```python
from build123d import *

# Parameters (mm, degrees)
BOSS_EXTRUDE1_DEPTH = 5
CUT_EXTRUDE1_REACH  = 7
SKETCH3_W           = 5
SKETCH3_H           = 26.5


with BuildPart() as part:
    # Sketch2 → Boss-Extrude1 (new body)
    with BuildSketch(Plane.XY):
        Polygon((-50, 422.98), (-50, 0), (50, 0), (50, 422.98), (50, 493.000753821), align=None)
    extrude(amount=BOSS_EXTRUDE1_DEPTH)

    # Sketch3 → Cut-Extrude1 (cut, up to next)
    with BuildSketch(Plane.XY.offset(5), mode=Mode.PRIVATE) as cut_extrude1_sk1:
        with Locations((42.5, 325)):
            Rectangle(SKETCH3_W, SKETCH3_H)
    cut_extrude1_tool1 = extrude(cut_extrude1_sk1.sketch, amount=-CUT_EXTRUDE1_REACH, mode=Mode.PRIVATE) & part.part
    add(cut_extrude1_tool1.solids().sort_by_distance((42.5, 325, 5))[0], mode=Mode.SUBTRACT)


solid = part.part
```
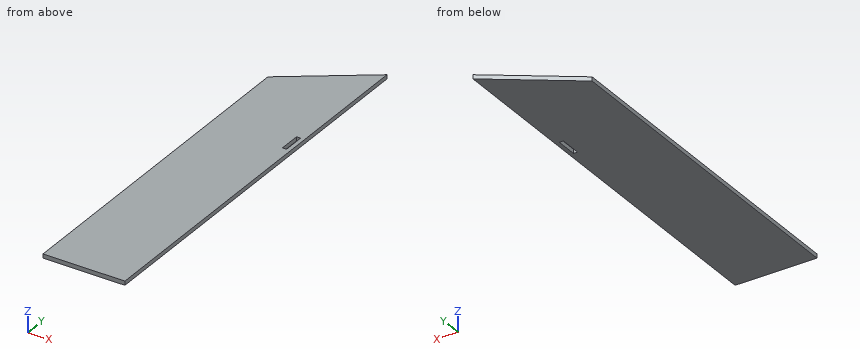
Could you check a few things on this model? Use its own coordinates, in mm. Give positions to 0.01 mm unless a question says otherwise; leave off trailing zeros. Loops run counter-clockwise (first coordinate to the right, second up) from the corner with the lowest first, then second, coordinate; pieces in that order, holes last. Notation, with made-up numbers: (22, 79.5) - (39, 79.5) arc R21 cw to (39, 90.5) - close; hole circle Ø5 at (24.25, -23). An arc over 180 degrees is marked (long way). Answer in a Markdown table with one row per item. Add a question column.
Q1. If we section it at A-A (y = 317.5): List the corners of the cut face in (x, z) for me.
Q2. If we section it at C-C (x = -32): List the corners of the cut face in (y, z) for me, plus the area to 3 significant figures.
Q3. If we section it at D-D (y = 444): List the corners of the cut face in (x, z) for me.
Q4. For pin 1 (8 mm diameter, centred on x = 34.5, y = 318.5, fed in from -Z); pin 2 (3 mm diameter, centred on x = -6, z = 3.5, fed in from +Y), each with a flat end and sliding along its axis, tell me the tip position at first contact or that it passes through.
Q5. If we section it at B-B (z = 3.85): List the corners of the cut face in (x, y) for me, plus the area to 3 significant figures.
Q6. Please list where these lines run through material, in increasing order: L1, parallel to X at y = 438, z = 1.75; L2, parallel to X at y = 469.5, z = 3.45; L3, parallel to Y at x = -4.5, z = 2.45. Write a range as from..to.
The answers:
| question | item | result |
|---|---|---|
| 1 | outline | (-50, 0) - (40, 0) - (40, 5) - (-50, 5) - close; (45, 0) - (50, 0) - (50, 5) - (45, 5) - close |
| 2 | outline | (0, 0) - (435.58, 0) - (435.58, 5) - (0, 5) - close |
| 2 | area | 2,180 mm^2 |
| 3 | outline | (-19.98, 0) - (50, 0) - (50, 5) - (-19.98, 5) - close |
| 4 | pin 1 | stops at z = 0 |
| 4 | pin 2 | stops at y = 454.84 |
| 5 | outline | (-50, 0) - (50, 0) - (50, 493) - (-50, 422.98) - close; hole (40, 311.75) - (45, 311.75) - (45, 338.25) - (40, 338.25) - close |
| 5 | area | 45,700 mm^2 |
| 6 | L1 | x = -28.55..50 |
| 6 | L2 | x = 16.44..50 |
| 6 | L3 | y = 0..454.84 |
